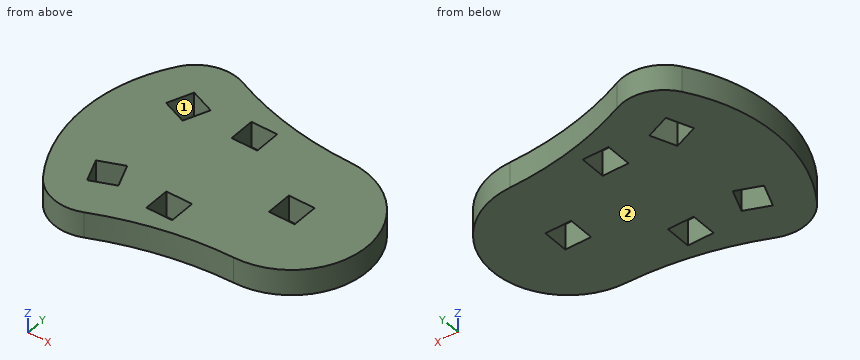
from build123d import *

# Parameters (mm, degrees)
SKETCH1_W           = 1.524
SKETCH1_H           = 1.524
BOSS_EXTRUDE1_DEPTH = 1.524


with BuildPart() as part:
    # Sketch1 → Boss-Extrude1 (new body)
    with BuildSketch(Plane.XY):
        with BuildLine():
            ThreePointArc((-3.625849071, -6.846112432), (-5.351927636, -6.959401294), (-6.750279516, -5.941170673))
            ThreePointArc((-6.750279516, -5.941170673), (-8.335255099, -0.762), (-6.750279516, 4.417170673))
            ThreePointArc((-6.750279516, 4.417170673), (-5.351927636, 5.435401294), (-3.625849071, 5.322112432))
            ThreePointArc((-3.625849071, 5.322112432), (0.088431716, 4.124975631), (3.96754689, 3.69896653))
            ThreePointArc((3.96754689, 3.69896653), (8.42851342, -0.762), (3.96754689, -5.22296653))
            ThreePointArc((3.96754689, -5.22296653), (0.088431716, -5.648975631), (-3.625849071, -6.846112432))
        make_face()
        with Locations((-0.762, -4.025750638)):
            Rectangle(SKETCH1_W, SKETCH1_H, mode=Mode.SUBTRACT)
        with Locations((-0.762, 2.501750638)):
            Rectangle(SKETCH1_W, SKETCH1_H, mode=Mode.SUBTRACT)
        with Locations((3.96754689, -0.762)):
            Rectangle(SKETCH1_W, SKETCH1_H, mode=Mode.SUBTRACT)
        Polygon((-5.542485833, 1.929853233), (-4.970674394, 3.342513022), (-3.558014606, 2.770701583), (-4.129826044, 1.358041795), align=None, mode=Mode.SUBTRACT)
        Polygon((-4.129826044, -2.882041795), (-5.542485833, -3.453853233), (-4.970674394, -4.866513022), (-3.558014606, -4.294701583), align=None, mode=Mode.SUBTRACT)
    extrude(amount=-BOSS_EXTRUDE1_DEPTH)


solid = part.part
Read the model definition and answer for the solid it produces. Units are mm, in the model's axes. Face numbers are marked on the shaded views. A direction names the side the tool comes from. Coordinates: 2 decimals unless noted, no trailing zeros. Order: outer loops, then holes, each group sorted by start corner. A loop starts at its lowest first (then second) coordinate and runs counter-clockwise, first axis right, second up. Notation, with made-up numbers: (47, -23.75) -> (94, -23.75) arc R25 ccw to (94, 2.25) -> close; hole circle Ø4 at (48.25, -24). An arc over 180 degrees is marked (long way). Answer as a JSON object with one key per item and string values.
1) A cutting plane is placed at D-D, the plane y = -1. Determine the outline of the cut face in (x, z), plus the area to 3 significant figures.
Model answer:
{"outline": "(-8.33, -1.52) -> (3.21, -1.52) -> (3.21, 0) -> (-8.33, 0) -> close; (4.73, -1.52) -> (8.42, -1.52) -> (8.42, 0) -> (4.73, 0) -> close", "area": "23.2 mm²"}
2) Each of these flat-tipped pins is pushed along its axis until it touches: pin 1 (0.5 mm diameter, centred on x = -1, z = -0.5, fed in from +Y); pin 2 (0.5 mm diameter, centred on x = 3.5, z = -1, fed in from -Y); pin 3 (0.5 mm diameter, centred on y = -4, z = -1, fed in from -X). Where does it stop, or does it pass through?
Model answer:
{"pin 1": "stops at y = 4.46", "pin 2": "stops at y = -5.24", "pin 3": "stops at x = -7.84"}
3) A cutting plane is placed at C-C, the plane x = -0.75. Determine the outline of the cut face in (y, z), plus the area to 3 significant figures.
Model answer:
{"outline": "(-5.85, -1.52) -> (-4.79, -1.52) -> (-4.79, 0) -> (-5.85, 0) -> close; (-3.26, -1.52) -> (1.74, -1.52) -> (1.74, 0) -> (-3.26, 0) -> close; (3.26, -1.52) -> (4.32, -1.52) -> (4.32, 0) -> (3.26, 0) -> close", "area": "10.9 mm²"}
4) A tool of negligible diameter and unlimited length cuts with its end or side. For the marked faces 1 and 2, from which of +Z, -Z, +X, -X, +Y, -Y can it reach the whole face along a straight path? Write none if from no direction.
Model answer:
{"face 1": "+Z, -Z", "face 2": "-Z, +X, -X, +Y, -Y"}
5) A cutting plane is placed at B-B, the plane y = -4.5. Determine the outline of the cut face in (x, z).
Model answer:
{"outline": "(-7.55, -1.52) -> (-5.12, -1.52) -> (-5.12, 0) -> (-7.55, 0) -> close; (-4.07, -1.52) -> (-1.52, -1.52) -> (-1.52, 0) -> (-4.07, 0) -> close; (0, -1.52) -> (6.4, -1.52) -> (6.4, 0) -> (0, 0) -> close"}
6) Consider line 1 along Y through (x, z) = (-5.25, -0.5); line 2 along Y through (x, z) = (4, -0.9); line 3 along X through (y, z) = (2.5, -0.65). Determine where each line is inside the solid, lowest interval first. Write a range as from..to.
Model answer:
{"line 1": "y = -6.99..-4.18, -3.34..1.81, 2.65..5.46", "line 2": "y = -5.22..-1.52, 0..3.7", "line 3": "x = -7.74..-5.31, -3.67..-1.52, 0..7.01"}
7) A cutting plane is placed at A-A, the plane z = -0.9. Determine the outline of the cut face in (x, y), plus the area to 3 significant figures.
Model answer:
{"outline": "(-6.75, -5.94) arc R2.54 ccw to (-3.63, -6.85) arc R19.31 cw to (3.97, -5.22) arc R4.46 ccw to (3.97, 3.7) arc R19.31 cw to (-3.63, 5.32) arc R2.54 ccw to (-6.75, 4.42) arc R9.25 ccw to start; hole (-5.54, -3.45) -> (-4.97, -4.87) -> (-3.56, -4.29) -> (-4.13, -2.88) -> close; hole (-5.54, 1.93) -> (-4.13, 1.36) -> (-3.56, 2.77) -> (-4.97, 3.34) -> close; hole (-1.52, -4.79) -> (0, -4.79) -> (0, -3.26) -> (-1.52, -3.26) -> close; hole (-1.52, 1.74) -> (0, 1.74) -> (0, 3.26) -> (-1.52, 3.26) -> close; hole (3.21, -1.52) -> (4.73, -1.52) -> (4.73, 0) -> (3.21, 0) -> close", "area": "145 mm²"}
